```python
from build123d import *

# Parameters (mm, degrees)
SKETCH1_R           = 5
BOSS_EXTRUDE1_DEPTH = 5


with BuildPart() as part:
    # Sketch1 → Boss-Extrude1 (new body)
    with BuildSketch(Plane(origin=(0, 0, 0), x_dir=(1, 0, 0), z_dir=(0, 1, 0))):
        with BuildLine():
            Line((49, -62.104477612), (-181, -62.104477612))
            ThreePointArc((-181, -62.104477612), (-188.071067812, -59.175545424), (-191, -52.104477612))
            Line((-191, -52.104477612), (-191, -17.104477612))
            Line((-191, -17.104477612), (-128, -17.104477612))
            Line((-128, -17.104477612), (-128, -2.104477612))
            Line((-128, -2.104477612), (-191, -2.104477612))
            Line((-191, -2.104477612), (-191, 32.895522388))
            ThreePointArc((-191, 32.895522388), (-188.071067812, 39.9665902), (-181, 42.895522388))
            Line((-181, 42.895522388), (49, 42.895522388))
            Line((49, 42.895522388), (141, 20.395522388))
            Line((141, 20.395522388), (191, 20.395522388))
            Line((191, 20.395522388), (191, -39.604477612))
            Line((191, -39.604477612), (141, -39.604477612))
            Line((141, -39.604477612), (49, -62.104477612))
        make_face()
        with Locations(Location((167.053731343, -9.604477612, 0), (0, 0, 270))):
            Circle(SKETCH1_R, mode=Mode.SUBTRACT)
    extrude(amount=BOSS_EXTRUDE1_DEPTH)


solid = part.part
```
Work out the finished part from the listing and answer in its coordinate system (mm). Round coordinates to 2 decimals unless told otherwise and drop trailing zeros. Write each loop counter-clockwise with the first axis right and the second up, starting at its lowest first coordinate (ties: lowest second). Pieces come first, ordered by that corner, then holes. Notation, with made-up numbers: (57, 2) -> (87, 2) arc R16 cw to (87, 6) -> close; hole circle Ø5 at (47.5, 56.5). An arc over 180 degrees is marked (long way). Write each question's results on one line, items separated by ' | '.
1) The part is cut by section B-B (z = -25.5). Write down the section's boundary in (x, y).
Findings:
outline: (-191, 0) -> (120.13, 0) -> (120.13, 5) -> (-191, 5) -> close
2) For a pull along X with two mould halves and no side action, classify faces 1 (the cylindrical face through (162.173, 2.465, 8.521)), 2 (the cylindrical face through (-188.148, 2.465, -39.888)), 3 (the flat face through (3, 5, 9)), 4 (the flat face through (94.36, 2.46, -31.8)) as +X half, -X half, draft (parallel to the pull), parting line (faces both ways), or undercut.
Findings:
face 1: undercut | face 2: -X half | face 3: draft | face 4: +X half
3) Flat-ended cylindrical pins translate along their axes: pin 1 (2 mm diameter, centred on x = 127.5, y = 2, fed in from -Z); pin 2 (2.5 mm diameter, centred on x = 162.5, y = 1.5, fed in from +Z); pin 3 (1.5 mm diameter, centred on y = 3.5, z = 9, fed in from -X). Find the tip coordinate at first contact, or state that the pin passes through.
Findings:
pin 1: stops at z = -23.94 | pin 2: stops at z = 39.6 | pin 3: stops at x = -128
4) Consider line 1 along Z through (x, y) = (-152, 3.85); line 2 along X through (y, z) = (4.5, 2.5); line 3 along Z through (x, y) = (160, 2.25). Determine where each line is inside the solid, lowest interval first. Write a range as [from, to].
Findings:
line 1: z = [-42.9, 2.1], [17.1, 62.1] | line 2: x = [-128, 191] | line 3: z = [-20.4, 39.6]
5) The part is cut by section C-C (x = 90.5). Write down the section's boundary in (y, z), and give its area (3 significant figures).
Findings:
outline: (0, -32.75) -> (5, -32.75) -> (5, 51.96) -> (0, 51.96) -> close | area: 424 mm²
6) The part is cut by section A-A (y = 2.5). Write down the section's boundary in (x, z), and give its area (3 significant figures).
Findings:
outline: (-191, -32.9) arc R10 ccw to (-181, -42.9) -> (49, -42.9) -> (141, -20.4) -> (191, -20.4) -> (191, 39.6) -> (141, 39.6) -> (49, 62.1) -> (-181, 62.1) arc R10 ccw to (-191, 52.1) -> (-191, 17.1) -> (-128, 17.1) -> (-128, 2.1) -> (-191, 2.1) -> close; hole circle Ø10 at (167.05, 9.6) | area: 34,700 mm²
